Work out the finished part from the listing and answer in its coordinate system (mm). A direction names the side the tool comes from. Coordinates: 2 decimals unless noted, no trailing zeros. Use a Markdown table: item, result. Add a question column.
(1) For a pull along X with two mould halves and no side action, classify faces 3 (the face through (136.539, 454.346, 4.93)), 4 (the face through (110, 600, 10)), 5 (the face through (223, 296, 10)) as released by +X, released by -X, zero draft, split by the parting line, or undercut.
(2) Find the intervals of material crossed by line 1 (Y direction, x = 140, z = 16.5); line 2 (X direction, y = 460, z = 4.75); line 3 (Y direction, x = 140, z = 7), in increasing order. Write a range as from..to.
(3) A tool of negligible diameter and unlimited length cuts with its end or side. For faces 1 (the face through (135.968, 542.324, 4.93)), 2 (the face through (110, 0, 10)), from which of +Z, -Z, +X, -X, +Y, -Y can it reach the whole face along a straight path? Write none if from no direction.
(4) Given pin 1 Ø4.5 at (x, y) = (133, 183) entering from -Z, flat-ended and moving along its own axis, determine where the tip first touches the part or whether it passes through.
from build123d import *

# Parameters (mm, degrees)
SKETCH1_W                                           = 223
SKETCH1_H                                           = 600
BOSS_EXTRUDE1_DEPTH                                 = 20
CBORE_FOR_M6_HEX_SOCKET_HEAD_CAP_SCREW1_D           = 6.5
CBORE_FOR_M6_HEX_SOCKET_HEAD_CAP_SCREW1_CBORE_D     = 15
CBORE_FOR_M6_HEX_SOCKET_HEAD_CAP_SCREW1_CBORE_DEPTH = 10
CBORE_FOR_M6_HEX_SOCKET_HEAD_CAP_SCREW2_D           = 6.5
CBORE_FOR_M6_HEX_SOCKET_HEAD_CAP_SCREW2_CBORE_D     = 15
CBORE_FOR_M6_HEX_SOCKET_HEAD_CAP_SCREW2_CBORE_DEPTH = 10
SKETCH6_R                                           = 3.75
CUT_EXTRUDE1_DEPTH                                  = 641.413147898
M5_TAPPED_HOLE1_D                                   = 4.2
M5_TAPPED_HOLE1_DEPTH                               = 12.4
M5_TAPPED_HOLE1_TIP                                 = 1.2618073


with BuildPart() as part:
    # Sketch1 → Boss-Extrude1 (new body)
    with BuildSketch(Plane.XY):
        with Locations((111.5, 300)):
            Rectangle(SKETCH1_W, SKETCH1_H)
    extrude(amount=BOSS_EXTRUDE1_DEPTH)

    # CBORE for M6 Hex Socket Head Cap Screw1 (through all)
    with Locations(Plane(origin=(0, 0, 0), x_dir=(-1, 0, 0), z_dir=(0, 0, -1))):
        with Locations((-134.5, 115), (-134.5, 185), (-92, 107.5), (-92, 192.5)):
            CounterBoreHole(CBORE_FOR_M6_HEX_SOCKET_HEAD_CAP_SCREW1_D / 2, CBORE_FOR_M6_HEX_SOCKET_HEAD_CAP_SCREW1_CBORE_D / 2, CBORE_FOR_M6_HEX_SOCKET_HEAD_CAP_SCREW1_CBORE_DEPTH)

    # CBORE for M6 Hex Socket Head Cap Screw2 (through all)
    with Locations(Plane(origin=(0, 0, 0), x_dir=(-1, 0, 0), z_dir=(0, 0, -1))):
        with Locations((-87.5, 368.5), (-87.5, 553.5), (-140, 386), (-140, 461), (-140, 536)):
            CounterBoreHole(CBORE_FOR_M6_HEX_SOCKET_HEAD_CAP_SCREW2_D / 2, CBORE_FOR_M6_HEX_SOCKET_HEAD_CAP_SCREW2_CBORE_D / 2, CBORE_FOR_M6_HEX_SOCKET_HEAD_CAP_SCREW2_CBORE_DEPTH)

    # Sketch6 → Cut-Extrude1 (cut, through all)
    with BuildSketch(Plane.XY.offset(20)):
        with Locations((203, 460)):
            Circle(SKETCH6_R)
    extrude(amount=-CUT_EXTRUDE1_DEPTH, mode=Mode.SUBTRACT)

    # M5 Tapped Hole1
    with Locations(Plane.XY.offset(20)):
        with Locations((213, 590)):
            Hole(M5_TAPPED_HOLE1_D / 2, depth=M5_TAPPED_HOLE1_DEPTH)
            with Locations((0, 0, -(M5_TAPPED_HOLE1_DEPTH + M5_TAPPED_HOLE1_TIP / 2))):  # 118° drill point
                Cone(0, M5_TAPPED_HOLE1_D / 2, M5_TAPPED_HOLE1_TIP, mode=Mode.SUBTRACT)


solid = part.part
Model answer:
| question | item | result |
|---|---|---|
| 1 | face 3 | undercut |
| 1 | face 4 | zero draft |
| 1 | face 5 | released by +X |
| 2 | line 1 | 0..382.75, 389.25..457.75, 464.25..532.75, 539.25..600 |
| 2 | line 2 | 0..132.57, 147.43..199.25, 206.75..223 |
| 2 | line 3 | 0..109.9, 120.1..179.9, 190.1..378.5, 393.5..453.5, 468.5..528.5, 543.5..600 |
| 3 | face 1 | -Z |
| 3 | face 2 | +Z, -Z, +X, -X, -Y |
| 4 | pin 1 | z = 10 |
